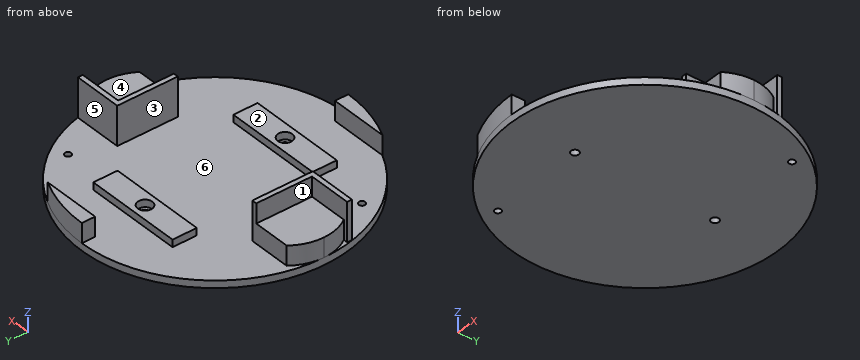
```python
from build123d import *

# Parameters (mm, degrees)
SKETCH_R        = 55
PAD_DEPTH       = 3
PAD001_DEPTH    = 16
PAD002_DEPTH    = 8
SKETCH003_R     = 1.3
POCKET_DEPTH    = 5
SKETCH004_W     = 40
SKETCH004_H     = 10
SKETCH004_R     = 1.6
PAD003_DEPTH    = 6
SKETCH005_R     = 3
POCKET001_DEPTH = 3
SKETCH006_R     = 1.6
POCKET002_DEPTH = 6
PAD004_DEPTH    = 8


with BuildPart() as part:
    # Sketch → Pad (new body)
    with BuildSketch(Plane.XY):
        Circle(SKETCH_R)
    extrude(amount=PAD_DEPTH)

    # Sketch001 (on Face3 of Pad) → Pad001 (join)
    with BuildSketch(Plane.XY.offset(3)):
        Polygon((33.500008, 0), (33.500008, 13), (53.345406, 13), (53.345406, 11), (35.5, 11), (35.5, -0.005684), (35.5, -12), (33.500008, -12), align=None)
        Polygon((-33.5, 0), (-33.5, -13), (-53.293575, -13), (-53.293575, -11), (-35.5, -11), (-35.5, 0.001212), (-35.5, 12), (-33.5, 12), align=None)
    extrude(amount=PAD001_DEPTH)

    # Sketch002 (on Face3 of Pad001) → Pad002 (join)
    with BuildSketch(Plane.XY.offset(3)):
        with BuildLine():
            ThreePointArc((-23.973944, -49.5), (-12.298374, -53.607369), (0, -55))
            Line((0, -49.5), (0, -55))
            Line((-23.973944, -49.5), (0, -49.5))
        make_face()
        with BuildLine():
            ThreePointArc((23.973944, 49.5), (12.298374, 53.607369), (0, 55))
            Line((0, 49.5), (0, 55))
            Line((23.973944, 49.5), (0, 49.5))
        make_face()
    extrude(amount=PAD002_DEPTH)

    # Sketch003 (on Face3 of Pad002) → Pocket (cut)
    with BuildSketch(Plane.XY.offset(3)):
        with Locations((-40, -28)):
            Circle(SKETCH003_R)
        with Locations((40, 28)):
            Circle(SKETCH003_R)
    extrude(amount=-POCKET_DEPTH, mode=Mode.SUBTRACT)

    # Sketch004 (on Face2 of Pocket) → Pad003 (join)
    with BuildSketch(Plane(origin=(0, 0, 0), x_dir=(1, 0, 0), z_dir=(0, 0, -1))):
        with Locations((0, -28.9)):
            Rectangle(SKETCH004_W, SKETCH004_H)
        with Locations((0, -28.9)):
            Circle(SKETCH004_R, mode=Mode.SUBTRACT)
        with Locations((0, 28.9)):
            Rectangle(SKETCH004_W, SKETCH004_H)
        with Locations((0, 28.9)):
            Circle(SKETCH004_R, mode=Mode.SUBTRACT)
    extrude(amount=-PAD003_DEPTH)

    # Sketch005 (on Face42 of Pad003) → Pocket001 (cut)
    with BuildSketch(Plane.XY.offset(6)):
        with Locations((0, 28.9)):
            Circle(SKETCH005_R)
        with Locations((0, -28.9)):
            Circle(SKETCH005_R)
    extrude(amount=-POCKET001_DEPTH, mode=Mode.SUBTRACT)

    # Sketch006 (on Face42 of Pocket001) → Pocket002 (cut)
    with BuildSketch(Plane.XY.offset(6)):
        with Locations((0, 28.9)):
            Circle(SKETCH006_R)
        with Locations((0, -28.9)):
            Circle(SKETCH006_R)
    extrude(amount=-POCKET002_DEPTH, mode=Mode.SUBTRACT)

    # Sketch007 (on Face3 of Pocket002) → Pad004 (join)
    with BuildSketch(Plane.XY.offset(3)):
        with BuildLine():
            Line((-35.5, 0), (-35.5, 12))
            Line((-35.5, 12), (-50.870426, 12))
            ThreePointArc((-50.870426, 12), (-53.938727, 6.34534), (-55, 0))
            ThreePointArc((-55, 0), (-54.130945, -5.756552), (-51.601242, -11))
            Line((-35.5, -11), (-51.601242, -11))
            Line((-35.5, 0), (-35.5, -11))
        make_face()
    pad004 = extrude(amount=PAD004_DEPTH)

    # Mirrored: Pad004 across Sketch007 V_Axis
    add(pad004.mirror(Plane(origin=(0, 0, 3), x_dir=(0, 0, 1), z_dir=(1, 0, 0))))


solid = part.part
```
The model under review builds one solid part; all positions refer to its coordinate system, in mm. Face numbers are marked on the shaded views. A direction names the side the tool comes from. Round coordinates to 2 decimals unless told otherwise and drop trailing zeros. Write each loop counter-clockwise with the first axis right and the second up, starting at its lowest first coordinate (ties: lowest second). Pieces come first, ordered by that corner, then holes. Notation, with made-up numbers: (-36, -37) - (-5, -37) arc R13 cw to (-5, -28) - close; hole circle Ø2 at (73.5, -30). An arc over 180 degrees is marked (long way). Answer as CSV lines item,"result". Start each with the question number.
(1) We need section A-A on z = 15.25. State the section outline as (x, y) points, plus the area to 3 significant figures.
(2) To check wall thickness, follow line 1 (Y direction, x = 0, z = 0.9); line 2 (Y direction, x = 5, z = 5.75); line 3 (X direction, y = -0.5, z = 18). State the ranges of each line that lie inside material, in increasing order.
(3) Draft analysis for pull direction Y (two halves, no side actions). For the marked faces 4, 5 and 6, state which applies: pulls with the +Y half, pulls with the -Y half, needs draft (parallel to the pull), parting line crosses it, or undercut.
(4) We need section B-B on x = 40. State the section outline as (y, z) points, plus the area to 3 significant figures.
(5) For pin 1 Ø5 at (x, y) = (-39, -9.5) entering from -Z; pin 2 Ø5 at (x, y) = (-7, 29) entering from +Z; pin 3 Ø3.5 at (x, y) = (-40, -28) entering from +Z; pin 4 Ø3 at (y, z) = (-51, 7.5) entering from +X, all flat-tipped, find the tip position at first contact; note any pin that passes through.
(6) For the marked faces 1, 2 and 3, list the 3-axis set-ups (+Z, -Z, +X, -X, +Y, -Y) from which the entire face can be reached by the end or side of a thin tool; tool diameter is ignored.
(7) We need section C-C on z = 9.5. State the section outline as (x, y) points, plus the area to 3 significant figures.
Worked answers:
1,outline,"(-53.29, -13) - (-33.5, -13) - (-33.5, 12) - (-35.5, 12) - (-35.5, -11) - (-53.29, -11) - close; (33.5, -12) - (35.5, -12) - (35.5, 11) - (53.35, 11) - (53.35, 13) - (33.5, 13) - close"
1,area,"171 mm²"
2,line 1,"-55 to -30.5, -27.3 to 27.3, 30.5 to 55"
2,line 2,"-33.9 to -23.9, 23.9 to 33.9, 49.5 to 54.77"
2,line 3,"-35.5 to -33.5, 33.5 to 35.5"
3,face 4,"needs draft"
3,face 5,"pulls with the +Y half"
3,face 6,"undercut"
4,outline,"(-37.75, 0) - (26.7, 0) - (26.7, 3) - (13, 3) - (13, 19) - (11, 19) - (11, 11) - (-11, 11) - (-11, 3) - (-37.75, 3) - close; (29.3, 0) - (37.75, 0) - (37.75, 3) - (29.3, 3) - close"
4,area,"427 mm²"
5,pin 1,"z = 0"
5,pin 2,"z = 6"
5,pin 3,"z = 3"
5,pin 4,"x = 0"
6,face 1,"+Z, -X, +Y"
6,face 2,"+Z, +X, -X"
6,face 3,"+Z, +Y, -Y"
7,outline,"(-55, 0) arc R19.5 ccw to (-51.6, -11) - (-53.29, -11) - (-53.29, -13) - (-33.5, -13) - (-33.5, 12) - (-50.87, 12) arc R19.5 ccw to start; (-23.97, -49.5) arc R55 ccw to (0, -55) - (0, -49.5) - close; (0, 49.5) - (23.97, 49.5) arc R55 ccw to (0, 55) - close; (33.5, -12) - (35.5, -12) - (35.5, -11) - (51.6, -11) arc R19.5 ccw to (55, 0) arc R19.5 ccw to (51.6, 11) - (53.35, 11) - (53.35, 13) - (33.5, 13) - close"
7,area,"1,170 mm²"
